Build history of the part. All positions in model axes, mm. A direction names the side the tool comes from. Give positions to 0.01 mm unless a question says otherwise; leave off trailing zeros. Loops run counter-clockwise (first coordinate to the right, second up) from the corner with the lowest first, then second, coordinate; pieces in that order, holes last. Notation, with made-up numbers: M 24,-5.5 L 53,-5.5 A8 cw 53,8.5 Z; hole C 54,-13 d8. An arc over 180 degrees is marked long. Put each result on its own line as item: value.
Autodesk Inventor part; units mm, degrees
ref_plane "YZ Plane" through (0, 0, 0) normal (1, 0, 0) x (0, 1, 0)
ref_plane "XZ Plane" through (0, 0, 0) normal (0, 1, 0) x (-1, 0, 0)
ref_plane "XY Plane" through (0, 0, 0) normal (0, 0, 1) x (1, 0, 0)
sketch "Sketch1" plane through (0, 0, 0) normal (0, 1, 0) x (-1, 0, 0)
  line L0 (0, 0) -> (20, 0)
  line L1 (20, 0) -> (20, -2)
  line L2 (20, -2) -> (0, -2)
  line L3 (0, -2) -> (0, 0)
  dimension "d0" = 20
  dimension "d1" = 2
extrude "Extrusion1" add sketch "Sketch1" along normal blind 2
sketch "Sketch2" plane through (0, 2, 0) normal (0, 1, 0) x (1, 0, 0)
  line L0 (0, 2) -> (-20, 2)
  line L1 (0, 2) -> (0, 4)
  line L2 (0, 4) -> (2, 4)
  line L3 (2, 4) -> (2, -2)
  line L4 (2, -2) -> (0, -2)
  line L5 (0, 0) -> (0, 2)
  line L6 (0, -2) -> (0, 0)
  dimension "d4" = 2
  dimension "d5" = 2
  dimension "d6" = 6
extrude "Extrusion2" add sketch "Sketch2" against normal blind 2
sketch "Sketch3" plane through (0, 2, 0) normal (0, 1, 0) x (1, 0, 0)
  line L0 (0, 0) -> (0, -2)
  line L1 (0, -2) -> (0, -1)
  line L2 (2, 4) -> (2, -2)
  line L3 (2, -2) -> (2, -0.5)
  line L4 (2, -0.5) -> (1, -0.5)
  circle A0 centre (1, -0.5) radius 0.5
  line L5 (2, 1) -> (1.5, 1)
  circle A1 centre (1, 2.5) radius 0.5
  dimension "d9" = 1.5
  dimension "d10" = 1
  dimension "d11" = 1
extrude "Extrusion3" cut sketch "Sketch3" against normal blind 2
sketch "Sketch4" plane through (0, 2, -4) normal (-1, 0, 0) x (0, 0, 1)
  line L0 (2, 0) -> (4, 0)
  line L1 (3, 0) -> (3, -2)
  line L2 (2, -2) -> (4, -2)
  circle A0 centre (3, -1) radius 1
  line L3 (2, -2) -> (2, 0)
  circle A1 centre (3, -1) radius 1.4142
extrude "Extrusion4" cut sketch "Sketch4" along normal blind 100 contours L0 A0 L3 | L3 A1 | L0 A1 L2 A0 | A0 L2 L3
ref_plane "Work Plane1" through (-14, 1, -1) normal (-1, 0, 0) x (0, 0, 1)
sketch "Sketch5" plane through (-14, 1, -1) normal (-1, 0, 0) x (0, 0, 1)
  circle A0 centre (0, 0) radius 5
  point P0 (1, -1)
  dimension "d17" = 10
extrude "Extrusion5" add sketch "Sketch5" along normal mid plane 1
sketch "Sketch6" plane through (-20, 1, -1) normal (-1, 0, 0) x (0, 0, 1)
  circle A0 centre (0, 0) radius 5
  point P0 (1, -1)
extrude "Extrusion6" cut sketch "Sketch6" against normal blind 5.5
properties part number "drive_shaft"
Q1. Mould opens along Z. For faces 1 (the cylindrical face through (1, 1, 0)), 2 (the cylindrical face through (-14, 4, -5)), 3 (the flat face through (1, 1, -4)), 4 (the flat face through (0, 1, 1)) say: pulls with the +Z half, pulls with the -Z half, needs draft (parallel to the pull), parting line crosses it, or undercut.
Here are the results:
face 1: undercut
face 2: parting line crosses it
face 3: pulls with the -Z half
face 4: needs draft
Q2. Slice it at D-D (z = 1.75). List the corners of the cut face in (x, y).
Here are the results:
outline: M -14.5,-3.18 L -13.5,-3.18 L -13.5,5.18 L -14.5,5.18 Z; M 0,0 L 2,0 L 2,2 L 0,2 Z
Q3. Probe line 1 (Z direction, x = 1, y = 1.4); line 2 (X direction, y = 0.95, z = 0.5); line 3 (Z direction, x = -13.25, y = 1). List the from-to ranges inside material, lowest first. Write a range as from..to.
Here are the results:
line 1: -4..-3, -2..0, 1..2
line 2: -14.5..-13.5, 0..0.5, 1.5..2
line 3: -2..0
Q4. Slice it at B-B (y = 1). List the corners of the cut face in (x, z), and give its area (3 significant figures).
Here are the results:
outline: M -14.5,-6 L -13.5,-6 L -13.5,-2 L 0,-2 L 0,-4 L 2,-4 L 2,2 L 0,2 L 0,0 L -13.5,0 L -13.5,4 L -14.5,4 Z; hole C 1,-2.5 d1; hole C 1,0.5 d1
area: 47.4 mm²
Q5. Slice it at A-A (x = 1). List the corners of the cut face in (y, z).
Here are the results:
outline: M 0,-4 L 2,-4 L 2,-3 L 0,-3 Z; M 0,-2 L 2,-2 L 2,0 L 0,0 Z; M 0,1 L 2,1 L 2,2 L 0,2 Z
Q6. Slice it at C-C (z = -2.5). List the corners of the cut face in (x, y).
Here are the results:
outline: M -14.5,-3.77 L -13.5,-3.77 L -13.5,5.77 L -14.5,5.77 Z; M 0,0 L 0.5,0 L 0.5,2 L 0,2 Z; M 1.5,0 L 2,0 L 2,2 L 1.5,2 Z
Q7. Drop flat-ended pins along their axis: pin 1 Ø4 at (y, z) = (-2.5, -1.5) entering from +X; pin 2 Ø6 at (x, z) = (-1.5, -4.5) entering from +Y; pin 3 Ø0.6 at (x, y) = (1, 1.5) entering from -Z; pin 4 Ø4 at (x, z) = (-2, 3) entering from +Y. Give the stop position or say it passes through.
Here are the results:
pin 1: x = -13.5
pin 2: y = 2
pin 3: z = -4
pin 4: through
Q8. Tool access for faces 5 (the flat face through (1, 2, -1)), 6 (the flat face through (1, 1, 2)), 7 (the cylindrical face through (-7, 1, -2)): list every direction of +Z, -Z, +X, -X, +Y, -Y with a clear straight run to the whole face (end or side of a thin tool).
Here are the results:
face 5: +Z, -Z, +X, +Y
face 6: +Z, +X, +Y, -Y
face 7: none
